Part model, mm, in its own coordinate system. A direction names the side the tool comes from. Give positions to 0.01 mm unless a question says otherwise; leave off trailing zeros. Order: outer loops, then holes, each group sorted by start corner. A loop starts at its lowest first (then second) coordinate and runs counter-clockwise, first axis right, second up. Notation, with made-up numbers: (62.25, 82) -> (113.25, 82) arc R11 ccw to (113.25, 89) -> close; hole circle Ø3 at (3.5, 17). An arc over 180 degrees is marked (long way). Write item = value, one per line. Start each with the question number.
(1) Flat gauge pins, fed straight in: pin 1 (3.5 mm diameter, centred on x = 16.5, y = 4, fed in from -Z); pin 2 (1.5 mm diameter, centred on x = 14, z = -9.5, fed in from -Y); pin 3 (3.5 mm diameter, centred on x = 5.5, y = 11, fed in from -Z). Where does each tip first touch, or does it go through?
(2) Two-plate mould, pull along X, no slides. Class faces 4 (the cylindrical face through (0.285, 0.301, -4.549)), 5 (the flat face through (11, 15, -10)), 6 (the cylindrical face through (20.715, 14.014, -19.699)), 7 (the flat face through (2.5, 3, -4)): pulls with the +X half, pulls with the -X half, needs draft (parallel to the pull), parting line crosses it, or undercut.
(3) Saw through at D-D, the plane y = 1.5. List the corners of the cut face in (x, z) (3 decimals).
(4) Saw through at B-B, the plane z = -15. List the corners of the cut face in (x, y), then the cut area to 3 significant figures.
(5) Saw through at A-A, the plane x = 6.5. List the corners of the cut face in (y, z) (3 decimals).
(6) Saw through at C-C, the plane x = 16. List the corners of the cut face in (y, z) (3 decimals), then the cut area to 4 significant figures.
(7) Which spindle directions (+Z, -Z, +X, -X, +Y, -Y) get a long thin tool onto all of the face, cutting with end or side? Do faces 1 (the flat face through (16, 8, -6.445)), 2 (the cylindrical face through (6.01, 13.99, -15.65)), 3 (the flat face through (11, 13, -14)). Say none if no direction does.
(8) Probe line 1 along X through (y, z) = (7.5, -5.25); line 2 along X through (y, z) = (14, -15); line 3 along Z through (x, y) = (7.75, 4.5) (3 decimals). List the from-to ranges inside material, lowest first. Write a range as from..to.
from build123d import *

# Parameters (mm, degrees)
SKETCH1_W              = 21
SKETCH1_H              = 8
MAINBODY_DEPTH         = 15
SKETCH3_W              = 6.6
SKETCH3_H              = 4.89
QRDCLEARANCE_DEPTH     = 12
SKETCH4_W              = 4.6
SKETCH4_H              = 4.89
VISIONTUNNEL_DEPTH     = 3
FILLET1_R              = 1
SKETCH5_W              = 21
SKETCH5_H              = 2
FASTENINGBRACKET_DEPTH = 12
FILLET2_R              = 1
M2_CLEARANCE_HOLE1_D   = 2.4


with BuildPart() as part:
    # Sketch1 → mainBody (new body)
    with BuildSketch(Plane(origin=(0, 0, 0), x_dir=(1, 0, 0), z_dir=(0, 1, 0))):
        with Locations((10.5, 4)):
            Rectangle(SKETCH1_W, SKETCH1_H)
    extrude(amount=MAINBODY_DEPTH)

    # Sketch3 → QRDClearance (cut)
    with BuildSketch(Plane(origin=(0, 15, 0), x_dir=(1, 0, 0), z_dir=(0, 1, 0))):
        with Locations((5.3, 4)):
            Rectangle(SKETCH3_W, SKETCH3_H)
    qrdclearance = extrude(amount=-QRDCLEARANCE_DEPTH, mode=Mode.SUBTRACT)

    # Sketch4 → visionTunnel (cut)
    with BuildSketch(Plane(origin=(0, 3, 0), x_dir=(1, 0, 0), z_dir=(0, 1, 0))):
        with Locations((5.3, 4)):
            Rectangle(SKETCH4_W, SKETCH4_H)
    visiontunnel = extrude(amount=-VISIONTUNNEL_DEPTH, mode=Mode.SUBTRACT)

    # socketMirror: QRDClearance, visionTunnel across plane
    add(qrdclearance.mirror(Plane.ZY.offset(-10.5)), mode=Mode.SUBTRACT)
    add(visiontunnel.mirror(Plane.ZY.offset(-10.5)), mode=Mode.SUBTRACT)

    # Fillet1
    fillet1_edges = [part.edges().sort_by_distance(p)[0] for p in [
        (21, 0, -4),
        (10.5, 0, 0),
        (0, 0, -4),
        (21, 7.5, 0),
        (0, 7.5, 0),
    ]]
    fillet(fillet1_edges, radius=FILLET1_R)

    # Sketch5 → fasteningBracket (add)
    with BuildSketch(Plane(origin=(0, 0, -8), x_dir=(-1, 0, 0), z_dir=(0, 0, -1))):
        with Locations((-10.5, 14)):
            Rectangle(SKETCH5_W, SKETCH5_H)
    extrude(amount=FASTENINGBRACKET_DEPTH)

    # Fillet2
    fillet2_edges = [part.edges().sort_by_distance(p)[0] for p in [
        (0, 14, -20),
        (21, 14, -20),
        (10.5, 13, -8),
    ]]
    fillet(fillet2_edges, radius=FILLET2_R)

    # M2 Clearance Hole1 (through all)
    with Locations(Plane(origin=(5, 15, -15), x_dir=(0, 0, 1), z_dir=(0, 1, 0))):
        with Locations((0, 0), (0, 11)):
            Hole(M2_CLEARANCE_HOLE1_D / 2)


solid = part.part
Results list:
q1.pin_1 = -8
q1.pin_2 = 12.97
q1.pin_3 = -8.34
q2.face_4 = pulls with the -X half
q2.face_5 = needs draft
q2.face_6 = pulls with the +X half
q2.face_7 = undercut
q3.outline = (0, -8) -> (21, -8) -> (21, -1) arc R1 ccw to (20, 0) -> (1, 0) arc R1 ccw to (0, -1) -> close; hole (3, -6.445) -> (7.6, -6.445) -> (7.6, -1.555) -> (3, -1.555) -> close; hole (13.4, -6.445) -> (18, -6.445) -> (18, -1.555) -> (13.4, -1.555) -> close
q4.outline = (0, 13) -> (3.8, 13) -> (3.8, 15) -> (0, 15) -> close; (6.2, 13) -> (14.8, 13) -> (14.8, 15) -> (6.2, 15) -> close; (17.2, 13) -> (21, 13) -> (21, 15) -> (17.2, 15) -> close
q4.area = 32.4 mm^2
q5.outline = (0, -8) -> (12, -8) arc R1 cw to (13, -9) -> (13, -20) -> (15, -20) -> (15, -6.445) -> (0, -6.445) -> close; (0, -1.555) -> (15, -1.555) -> (15, 0) -> (1, 0) arc R1 ccw to (0, -1) -> close
q6.outline = (0, -8) -> (12, -8) arc R1 cw to (13, -9) -> (13, -13.8) -> (15, -13.8) -> (15, -6.445) -> (0, -6.445) -> close; (0, -1.555) -> (15, -1.555) -> (15, 0) -> (1, 0) arc R1 ccw to (0, -1) -> close; (13, -20) -> (15, -20) -> (15, -16.2) -> (13, -16.2) -> close
q6.area = 65.85 mm^2
q7.face_1 = +Y
q7.face_2 = +Y, -Y
q7.face_3 = -Z, +X, -X, -Y
q8.line_1 = 0..2, 8.6..12.4, 19..21
q8.line_2 = 0..3.8, 6.2..14.8, 17.2..21
q8.line_3 = -8..-6.445, -1.555..0
